Check sheet for the modelled part. Datum: model origin and axes. Units: mm. A direction names the side the tool comes from. Round coordinates to 2 decimals unless told otherwise and drop trailing zeros. Order: outer loops, then holes, each group sorted by start corner. A loop starts at its lowest first (then second) coordinate and runs counter-clockwise, first axis right, second up. Notation, with made-up numbers: (50, 53) -> (87, 53) arc R21 ccw to (87, 86) -> close; hole circle Ø8 at (14, 21). An arc over 180 degrees is marked (long way). Use CSV: the item, a comma, the result in double quotes.
```python
from build123d import *

# Parameters (mm, degrees)
F0_W     = 360
F0_H     = 500
F0_W_2   = 300
F0_H_2   = 440
F1_DEPTH = 30
F2_R     = 15
F3_DEPTH = 20
F3_TAPER = -20


with BuildPart() as f1:
    # F0 (on Top) → F1 (new body)
    with BuildSketch(Plane.XY):
        Rectangle(F0_W, F0_H)
        Rectangle(F0_W_2, F0_H_2, mode=Mode.SUBTRACT)
    extrude(amount=F1_DEPTH)

    # F2 (on face) → F3 (join)
    with BuildSketch(Plane(origin=(0, 0, 0), x_dir=(1, 0, 0), z_dir=(0, 0, -1))):
        with Locations((-165, 235)):
            Circle(F2_R)
        with Locations((-165, -235)):
            Circle(F2_R)
        with Locations((165, 235)):
            Circle(F2_R)
        with Locations((165, -235)):
            Circle(F2_R)
    extrude(amount=F3_DEPTH, taper=F3_TAPER)


solid = f1.part
```
Q1. Sectioned sample at A-A, the plane x = -100. Enter the section's corners in (y, z).
Result sheet:
outline,"(-250, 0) -> (-220, 0) -> (-220, 30) -> (-250, 30) -> close; (220, 0) -> (250, 0) -> (250, 30) -> (220, 30) -> close"
Q2. Mould release check, pull along X, two halves, no side actions. Record for faces 4 (the face through (-180, -3, 15)), 5 (the face through (152.093, -225.103, -3.473)), 6 (the face through (-165, -235, -20)): pulls with the +X half, pulls with the -X half, needs draft (parallel to the pull), parting line crosses it, or undercut.
Result sheet:
face 4,"pulls with the -X half"
face 5,"undercut"
face 6,"needs draft"
Q3. Sectioned sample at B-B, the plane y = -144. Enter the section's corners in (x, z).
Result sheet:
outline,"(-180, 0) -> (-150, 0) -> (-150, 30) -> (-180, 30) -> close; (150, 0) -> (180, 0) -> (180, 30) -> (150, 30) -> close"
Q4. Sectioned sample at C-C, the plane z = 6. Enter the section's corners in (x, y).
Result sheet:
outline,"(-180, -250) -> (180, -250) -> (180, 250) -> (-180, 250) -> close; hole (-150, -220) -> (150, -220) -> (150, 220) -> (-150, 220) -> close"
Q5. Scan lines: L1, parallel to Y at x = -6, z = 1.5; L2, parallel to X at y = 175, z = 24.5; L3, parallel to Y at x = 157, z = 5. Record each from-to range of solid material in increasing order.
Result sheet:
L1,"y = -250 to -220, 220 to 250"
L2,"x = -180 to -150, 150 to 180"
L3,"y = -250 to 250"
Q6. Access from +Z, -Z, +X, -X, +Y, -Y to the whole of each face (thin tool, end or side, straight path). Record for faces 1 (the face through (-3, -250, 15)), 2 (the face through (152.093, 244.897, -3.473)), 3 (the face through (-150, -3, 15)).
Result sheet:
face 1,"+Z, +X, -X, -Y"
face 2,"none"
face 3,"+Z, -Z"
Q7. Go/stop test with flat-tipped pins: pin 1 (24 mm diameter, centred on x = -1, z = 12, fed in from +Y); pin 2 (6 mm diameter, centred on y = -22, z = 12, fed in from +X); pin 3 (2 mm diameter, centred on x = -110, z = 14.5, fed in from -Y). Record where each tip stops, or that it passes through.
Result sheet:
pin 1,"stops at y = 250"
pin 2,"stops at x = 180"
pin 3,"stops at y = -250"
